The model under review builds one solid part; all positions refer to its coordinate system, in mm. A direction names the side the tool comes from. Coordinates: 2 decimals unless noted, no trailing zeros. Loops run counter-clockwise (first coordinate to the right, second up) from the corner with the lowest first, then second, coordinate; pieces in that order, holes last. Notation, with made-up numbers: (15, 30.25) - (29, 30.25) arc R20 cw to (29, 61.25) - close; hole circle Ø10 at (79, -22). An arc over 180 degrees is marked (long way). Answer in a Markdown table with one row per item. Add a question column.
(1) We need section A-A on x = 32.16. Write out the cut boundary in (y, z).
(2) Mouldability with a two-part tool opening along Z and no side actions: class faces 1 (the cylindrical face through (3, 1, 11)), 2 (the flat face through (38, 3, 6.5)), 3 (the flat face through (40.729, 3, 12)) as +Z half, -Z half, draft (parallel to the pull), parting line (faces both ways), or undercut.
(3) We need section D-D on z = 16.75. Write out the cut boundary in (x, y), plus the area to 3 significant figures.
(4) For line 1 along Z through (x, y) = (32.16, 0.6); line 2 along Z through (x, y) = (2.25, 0.5); line 3 along X through (y, z) = (0.95, 21.75), list the stretches that pass through material, from the lowest coordinate up.
(5) Machinability: for faces 4 (the flat face through (38, 3, 17.5)), 5 (the flat face through (34.729, 3, 12)), 6 (the flat face through (21, 0, 12)), which of the approach directions +Z, -Z, +X, -X, +Y, -Y give a long, thin tool a straight path to every point of the face, cutting with its end or side? Answer none if there is none.
(6) We need section B-B on z = 12. Write out the cut boundary in (x, y), plus the area to 4 significant figures.
(7) For P1, Ø0.8, axis at x = 37.5, y = 2.5, coming from the +Z side; P2, Ø6, axis at x = 12, z = 18.5, coming from the +Y side; P3, Ø2, axis at y = 3, z = 13.5, coming from the +X side, all flat-tipped, find the tip position at first contact; note any pin that passes through.
(8) We need section C-C on x = 2.25. Write out the cut boundary in (y, z).
from build123d import *

# Parameters (mm, degrees)
SKETCH2_W           = 42
SKETCH2_H           = 24
SKETCH2_R           = 1.25
BOSS_EXTRUDE1_DEPTH = 1.5
SKETCH2_9_W         = 6
SKETCH2_9_H         = 11
BOSS_EXTRUDE2_DEPTH = 4


with BuildPart() as part:
    # Sketch2 → Boss-Extrude1 (new body)
    with BuildSketch(Plane(origin=(0, 0, 0), x_dir=(1, 0, 0), z_dir=(0, 1, 0))):
        with Locations((21, -12)):
            Rectangle(SKETCH2_W, SKETCH2_H)
        with Locations((32.16, -2.25)):
            Circle(SKETCH2_R, mode=Mode.SUBTRACT)
        with Locations((32.16, -21.75)):
            Circle(SKETCH2_R, mode=Mode.SUBTRACT)
        with Locations((2.25, -12)):
            Circle(SKETCH2_R, mode=Mode.SUBTRACT)
    extrude(amount=BOSS_EXTRUDE1_DEPTH)

    # Sketch2<9> → Boss-Extrude2 (add)
    with BuildSketch(Plane(origin=(0, 0, 0), x_dir=(1, 0, 0), z_dir=(0, 1, 0))):
        with Locations((37.7285084, -12)):
            Rectangle(SKETCH2_9_W, SKETCH2_9_H)
    extrude(amount=BOSS_EXTRUDE2_DEPTH)


solid = part.part
Outcome:
| question | item | result |
|---|---|---|
| 1 | outline | (0, 0) - (1.5, 0) - (1.5, 1) - (0, 1) - close; (0, 3.5) - (1.5, 3.5) - (1.5, 20.5) - (0, 20.5) - close; (0, 23) - (1.5, 23) - (1.5, 24) - (0, 24) - close |
| 2 | face 1 | undercut |
| 2 | face 2 | -Z half |
| 2 | face 3 | draft |
| 3 | outline | (0, 0) - (42, 0) - (42, 1.5) - (40.73, 1.5) - (40.73, 4) - (34.73, 4) - (34.73, 1.5) - (0, 1.5) - close |
| 3 | area | 78.0 mm² |
| 4 | line 1 | 0 to 1, 3.5 to 20.5, 23 to 24 |
| 4 | line 2 | 0 to 10.75, 13.25 to 24 |
| 4 | line 3 | 0 to 30.91, 33.41 to 42 |
| 5 | face 4 | +Z, +X, -X, +Y |
| 5 | face 5 | +Z, -Z, -X, +Y |
| 5 | face 6 | +Z, -Z, +X, -X, -Y |
| 6 | outline | (0, 0) - (1, 0) - (1, 1.5) - (0, 1.5) - close; (3.5, 0) - (42, 0) - (42, 1.5) - (40.73, 1.5) - (40.73, 4) - (34.73, 4) - (34.73, 1.5) - (3.5, 1.5) - close |
| 6 | area | 74.25 mm² |
| 7 | P1 | z = 17.5 |
| 7 | P2 | y = 1.5 |
| 7 | P3 | x = 40.73 |
| 8 | outline | (0, 0) - (1.5, 0) - (1.5, 10.75) - (0, 10.75) - close; (0, 13.25) - (1.5, 13.25) - (1.5, 24) - (0, 24) - close |
